For this review, take the finished solid that the model builds, in its own axes (mm). Face numbers are marked on the shaded views. A direction names the side the tool comes from. Coordinates: 2 decimals unless noted, no trailing zeros. Order: outer loops, then holes, each group sorted by start corner. A loop starts at its lowest first (then second) coordinate and runs counter-clockwise, first axis right, second up. Notation, with made-up numbers: (19, 41.5) -> (41, 41.5) arc R35 ccw to (41, 76.5) -> close; hole circle Ø9 at (-16.75, 88.25). An arc over 180 degrees is marked (long way). Return JSON: item names as keys, results as strings. Group by question number.
Item 1: Machinability: for the marked faces 1, 2, 3, 4 and 5, which of the approach directions +Z, -Z, +X, -X, +Y, -Y give a long, thin tool a straight path to every point of the face, cutting with its end or side? Answer none if there is none.
Item 2: For line 1 along Y through (x, z) = (0, 1.4); line 2 along Z through (x, y) = (13.75, 7.5); line 3 along Y through (x, z) = (0.5, 1.5), list the stretches that pass through material, from the lowest coordinate up.
Item 3: Take a section at B-B (x = 10.5). Write out the cut boundary in (y, z), then the cut area to 3 significant figures.
Item 4: Insertion check: pin 1 (6 mm diameter, centred on x = -1, y = 0.5, fed in from +Z); pin 2 (2 mm diameter, centred on y = 8, z = 17.5, fed in from -X); pin 3 (5 mm diameter, centred on x = 0, y = 14.47, fed in from +Z); pin 4 (6 mm diameter, centred on y = 8.5, z = 17.5, fed in from -X). Each pin has a flat end and moves straight along its axis. Give the tip position at first contact, or say it passes through.
Item 5: Take a section at D-D (x = 6). Write out the cut boundary in (y, z), then the cut area to 3 significant figures.
Item 6: Draft analysis for pull direction Y (two halves, no side actions). For the marked faces 6, 7, 8 and 9, state which applies: +Y half, -Y half, draft (parallel to the pull), parting line (faces both ways), or undercut.
```python
from build123d import *

# Parameters (mm, degrees)
F0_W     = 28
F0_H     = 34.4861291724
F1_DEPTH = 8
F0_R     = 2
F2_DEPTH = 4
F4_START = 10
F4_DEPTH = 7.9999894
F5_START = 14
F3_R     = 2
F5_DEPTH = 4


with BuildPart() as f1:
    # F0 (on Top) → F1 (new body)
    with BuildSketch(Plane.XY):
        with Locations((4, 7.2430645862)):
            Rectangle(F0_W, F0_H)
        Polygon((3.875, 2.2372322931), (3.875, -2.2372322931), (-0.1381988935, -4.4744645862), (-3.875, -2.2372322931), (-3.875, 2.2372322931), (-0.1381988935, 4.4744645862), align=None, mode=Mode.SUBTRACT)
        Polygon((3.875, 16.7116968793), (3.875, 12.2372322931), (0, 10), (-3.875, 12.2372322931), (-3.875, 16.7116968793), (0, 18.9489291724), align=None, mode=Mode.SUBTRACT)
    extrude(amount=F1_DEPTH)

    # F0 (on Top) → F2 (join)
    with BuildSketch(Plane.XY):
        Polygon((0, 10), (3.875, 12.2372322931), (3.875, 16.7116968793), (0, 18.9489291724), (-3.875, 16.7116968793), (-3.875, 12.2372322931), align=None)
        with Locations((0, 14.4744645862)):
            Circle(F0_R, mode=Mode.SUBTRACT)
        Polygon((-0.1381988935, -4.4744645862), (3.875, -2.2372322931), (3.875, 2.2372322931), (-0.1381988935, 4.4744645862), (-3.875, 2.2372322931), (-3.875, -2.2372322931), align=None)
        Circle(F0_R, mode=Mode.SUBTRACT)
    extrude(amount=F2_DEPTH)

    # F3 (on Right) → F4 (join)
    with BuildSketch(Plane.YZ.offset(F4_START)):
        Polygon((-10, 27.9999948), (-10, 0), (24.4861291724, 0), (24.4861291724, 27.9999948), (7.2430645862, 27.9999948), align=None)
        Polygon((2.7686, 18.0050948), (5.0058322931, 21.8800948), (9.4802968793, 21.8800948), (11.7175291724, 18.0050948), (9.4802968793, 14.1300948), (5.0058322931, 14.1300948), align=None, mode=Mode.SUBTRACT)
    extrude(amount=F4_DEPTH)

    # F3 (on Right) → F5 (join)
    with BuildSketch(Plane.YZ.offset(F5_START)):
        Polygon((9.4802968793, 21.8800948), (5.0058322931, 21.8800948), (2.7686, 18.0050948), (5.0058322931, 14.1300948), (9.4802968793, 14.1300948), (11.7175291724, 18.0050948), align=None)
        with Locations((7.2430645862, 18.0050948)):
            Circle(F3_R, mode=Mode.SUBTRACT)
    extrude(amount=F5_DEPTH)


solid = f1.part
```
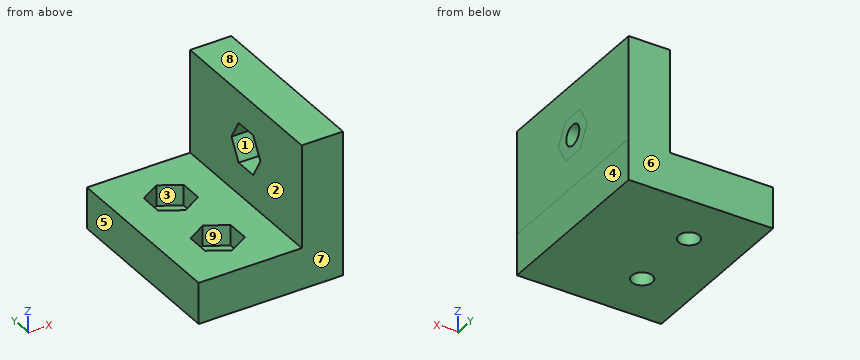
Findings below:
{
 "1": {"face 1": "-X", "face 2": "+Z, -X, +Y, -Y", "face 3": "+Z", "face 4": "+Z, -Z, +X, +Y, -Y", "face 5": "+Z, -Z, -X, +Y, -Y"},
 "2": {"line 1": "y = -10 to -2, 2 to 12.47, 16.47 to 24.49", "line 2": "z = 0 to 14.13, 21.88 to 28", "line 3": "y = -10 to -1.94, 1.94 to 12.54, 16.41 to 24.49"},
 "3": {"outline": "(-10, 0) -> (24.49, 0) -> (24.49, 28) -> (-10, 28) -> close; hole (2.77, 18.01) -> (5.01, 14.13) -> (9.48, 14.13) -> (11.72, 18.01) -> (9.48, 21.88) -> (5.01, 21.88) -> close", "area": "914 mm2"},
 "4": {"pin 1": "stops at z = 8", "pin 2": "passes through", "pin 3": "stops at z = 4", "pin 4": "stops at x = 10"},
 "5": {"outline": "(-10, 0) -> (24.49, 0) -> (24.49, 8) -> (-10, 8) -> close", "area": "276 mm2"},
 "6": {"face 6": "+Y half", "face 7": "-Y half", "face 8": "draft", "face 9": "undercut"}
}
